Model file for the job. Use its own axes, mm. A direction names the side the tool comes from. Give positions to 0.01 mm unless a question says otherwise; leave off trailing zeros. Loops run counter-clockwise (first coordinate to the right, second up) from the corner with the lowest first, then second, coordinate; pieces in that order, holes last. Notation, with made-up numbers: (68, 88) - (121, 88) arc R16 ccw to (121, 110) - close; hole circle Ø1 at (-9.5, 11). An arc over 180 degrees is marked (long way). Use a Markdown table: item, result.
from build123d import *

# Parameters (mm, degrees)
SKETCH_1_R      = 1.5
EXTRUDE_1_DEPTH = 2
SKETCH_3_W      = 43
SKETCH_3_H      = 40
SKETCH_3_R      = 1.75
EXTRUDE_2_DEPTH = 2


with BuildPart() as part:
    # 草图1 → 凸台-拉伸1 (new body)
    with BuildSketch(Plane(origin=(0, 0, 0), x_dir=(0, 0, -1), z_dir=(1, 0, 0))):
        with BuildLine():
            Line((-20, 0), (-20, -27))
            Line((-20, -27), (20, -27))
            Line((20, -27), (20, 0))
            ThreePointArc((20, 0), (0, 20), (-20, 0))
        make_face()
        with Locations((-15.5, 0)):
            Circle(SKETCH_1_R, mode=Mode.SUBTRACT)
        with Locations((-7.75, 13.423393759)):
            Circle(SKETCH_1_R, mode=Mode.SUBTRACT)
        with Locations((7.75, 13.423393759)):
            Circle(SKETCH_1_R, mode=Mode.SUBTRACT)
        with Locations((15.5, 0)):
            Circle(SKETCH_1_R, mode=Mode.SUBTRACT)
        with Locations((7.75, -13.423393759)):
            Circle(SKETCH_1_R, mode=Mode.SUBTRACT)
        with Locations((-7.75, -13.423393759)):
            Circle(SKETCH_1_R, mode=Mode.SUBTRACT)
        with BuildLine():
            Line((6.5, 7), (6.5, -7))
            ThreePointArc((6.5, -7), (0, -13.5), (-6.5, -7))
            Line((-6.5, -7), (-6.5, 7))
            ThreePointArc((-6.5, 7), (0, 13.5), (6.5, 7))
        make_face(mode=Mode.SUBTRACT)
    extrude(amount=EXTRUDE_1_DEPTH)

    # 草图3 → 凸台-拉伸2 (add)
    with BuildSketch(Plane.XZ.offset(27)):
        with Locations((21.5, 0)):
            Rectangle(SKETCH_3_W, SKETCH_3_H)
        with Locations(Location((9.5, 15, 0), (0, 0, 270))):
            Circle(SKETCH_3_R, mode=Mode.SUBTRACT)
        with Locations(Location((9.5, -15, 0), (0, 0, 270))):
            Circle(SKETCH_3_R, mode=Mode.SUBTRACT)
        with Locations(Location((33.5, 15, 0), (0, 0, 270))):
            Circle(SKETCH_3_R, mode=Mode.SUBTRACT)
        with Locations(Location((33.5, -15, 0), (0, 0, 270))):
            Circle(SKETCH_3_R, mode=Mode.SUBTRACT)
    extrude(amount=-EXTRUDE_2_DEPTH)


solid = part.part
(1) Mould opens along X. For faces 1 (the flat face through (43, -26, 0)), 2 (the cylindrical face through (34.026, -26.014, 13.331)), 3 (the cylindrical face through (1, -13.5, -0.1)), 4 (the cylindrical face through (34.026, -26.014, -16.669)) say: pulls with the +X half, pulls with the -X half, needs draft (parallel to the pull), parting line crosses it, or undercut.
Computed:
| item | result |
|---|---|
| face 1 | pulls with the +X half |
| face 2 | undercut |
| face 3 | needs draft |
| face 4 | undercut |
(2) 3-axis set-ups, long thin cutter, end or side, ignore diameter. For faces 5 (the cylindrical face through (1, 13.5, 0.1)), 6 (the flat face through (22, -25, 0)), 7 (the flat face through (15, -25.4, 20)): which of +Z, -Z, +X, -X, +Y, -Y reach the whole face in a straight line?
Computed:
| item | result |
|---|---|
| face 5 | +X, -X |
| face 6 | +Z, -Z, +X, +Y |
| face 7 | +Z, +X, -X, +Y, -Y |
(3) Drill centre lines: probe 1 along X at (y, z) = (-25.8, 15); probe 2 along Y at (x, z) = (1.4, 7.75); probe 3 along Y at (x, z) = (5, 0). Where is each one in solid material? Low to high. Write a range as [from, to].
Computed:
| item | result |
|---|---|
| probe 1 | [0, 7.75], [11.25, 31.75], [35.25, 43] |
| probe 2 | [-27, -14.92], [-11.92, 11.92], [14.92, 18.44] |
| probe 3 | [-27, -25] |
(4) Slice it at A-A, the plane z = 0. Write the cut outline in (x, y), plus the area to 3 significant figures.
Computed:
| item | result |
|---|---|
| outline | (0, -27) - (43, -27) - (43, -25) - (2, -25) - (2, -13.5) - (0, -13.5) - close; (0, 13.5) - (2, 13.5) - (2, 20) - (0, 20) - close |
| area | 122 mm² |
(5) Slice it at B-B, the plane y = -6. Write the cut outline in (x, z), plus the area to 3 significant figures.
Computed:
| item | result |
|---|---|
| outline | (0, -20) - (2, -20) - (2, -6.5) - (0, -6.5) - close; (0, 6.5) - (2, 6.5) - (2, 20) - (0, 20) - close |
| area | 54.0 mm² |
(6) Slice it at C-C, the plane x = 9.5. Write the cut outline in (y, z).
Computed:
| item | result |
|---|---|
| outline | (-27, -20) - (-25, -20) - (-25, -16.75) - (-27, -16.75) - close; (-27, -13.25) - (-25, -13.25) - (-25, 13.25) - (-27, 13.25) - close; (-27, 16.75) - (-25, 16.75) - (-25, 20) - (-27, 20) - close |
(7) Pin check, flat tips, straight feed: P1, Ø1, axis at y = -2.5, z = -10.5, coming from the +X side; P2, Ø2, axis at x = 33.5, z = 15, coming from the +Y side; P3, Ø4.5, axis at x = 33.5, z = -15, coming from the +Y side. Stop position of each tip, or through.
Computed:
| item | result |
|---|---|
| P1 | x = 2 |
| P2 | through |
| P3 | y = -25 |
(8) Slice it at D-D, the plane z = -15. Write the cut outline in (x, y), plus the area to 3 significant figures.
Computed:
| item | result |
|---|---|
| outline | (0, -27) - (7.75, -27) - (7.75, -25) - (2, -25) - (2, -1.41) - (0, -1.41) - close; (0, 1.41) - (2, 1.41) - (2, 13.23) - (0, 13.23) - close; (11.25, -27) - (31.75, -27) - (31.75, -25) - (11.25, -25) - close; (35.25, -27) - (43, -27) - (43, -25) - (35.25, -25) - close |
| area | 143 mm² |
